Can you work these out from the model? Positions are in its coordinate system, mm. Face numbers are marked on the shaded views. A direction names the side the tool comes from. Round coordinates to 2 decimals unless told otherwise and drop trailing zeros. Loops run counter-clockwise (first coordinate to the right, second up) from the corner with the lowest first, then second, coordinate; pieces in that order, holes last. Notation, with made-up numbers: (50.5, -26) -> (105.5, -26) arc R25 ccw to (105.5, -3) -> close; hole circle Ø6 at (-19, 1). An arc over 180 degrees is marked (long way). Write item = value, one per line.
from build123d import *

# Parameters (mm, degrees)
F1_DEPTH = 5
F2_R     = 1
F3_DEPTH = 25
F4_R     = 1
F5_DEPTH = 25
F6_R     = 4.99999
F7_R     = 5


# Not quite as in the source:
# - a fillet or chamfer is up to 0.001 mm smaller than in the source, because OpenCascade refuses the exact size
# - a feature names something its author has since deleted; it is built from what else it names


with BuildPart() as f1:
    # F0 (on Front) → F1 (new body, symmetric)
    with BuildSketch(Plane.XZ):
        with BuildLine():
            ThreePointArc((3.9053168747, -3.2800152603), (2.1542889978, -4.62266578), (0, -5.1))
            Line((0, -5.1), (0, -8))
            ThreePointArc((0, -8), (3.7724872299, -7.0546679653), (6.6534112025, -4.4420850251))
            Line((6.6534112025, -4.4420850251), (3.9053168747, -3.2800152603))
        make_face()
        with BuildLine():
            ThreePointArc((5.0737374807, -0.5169022898), (4.6972920498, -1.9863150301), (3.9053168747, -3.2800152603))
            Line((3.9053168747, -3.2800152603), (6.6534112025, -4.4420850251))
            ThreePointArc((6.6534112025, -4.4420850251), (7.3683012546, -3.1157882825), (7.8218318085, -1.6789720546))
            Line((7.8218318085, -1.6789720546), (5.0737374807, -0.5169022898))
        make_face()
        with BuildLine():
            ThreePointArc((2, 4.6914816423), (4.392181267, 2.5920539573), (5.0737374807, -0.5169022898))
            Line((5.0737374807, -0.5169022898), (7.8218318085, -1.6789720546))
            ThreePointArc((7.8218318085, -1.6789720546), (7.5363895919, 2.683809218), (5, 6.2449979984))
            ThreePointArc((5, 6.2449979984), (3.5795567819, 7.1544932207), (2, 7.7459666924))
            Line((2, 7.7459666924), (2, 4.6914816423))
        make_face()
        with BuildLine():
            ThreePointArc((7.8218318085, -1.6789720546), (7.3683012546, -3.1157882825), (6.6534112025, -4.4420850251))
            Line((6.6534112025, -4.4420850251), (18.8496842561, -9.5994480802))
            Line((18.8496842561, -9.5994480802), (20.018104862, -6.8363351098))
            Line((20.018104862, -6.8363351098), (7.8218318085, -1.6789720546))
        make_face()
        with BuildLine():
            Line((2, 15), (2, 7.7459666924))
            ThreePointArc((2, 7.7459666924), (3.5795567819, 7.1544932207), (5, 6.2449979984))
            Line((5, 6.2449979984), (5, 15))
            Line((5, 15), (2, 15))
        make_face()
    extrude(amount=F1_DEPTH, both=True)

    # F2 (on face) → F3 (cut)
    with BuildSketch(Plane(origin=(0.584210303, 0, 1.3815564852), x_dir=(0.9210376568, 0, -0.3894735353), z_dir=(0.3894735353, 0, 0.9210376568))):
        with Locations((16.1, 0)):
            Circle(F2_R)
    extrude(amount=-F3_DEPTH, mode=Mode.SUBTRACT)

    # F4 (on face) → F5 (cut)
    with BuildSketch(Plane.YZ.offset(5)):
        with Locations((0, 10.6224989992)):
            Circle(F4_R)
    extrude(amount=-F5_DEPTH, mode=Mode.SUBTRACT)

    # F6 (radius 5 in the source; OpenCascade refuses exactly that, so slightly less here)
    f6_edges = [f1.edges().sort_by_distance(p)[0] for p in [
        (19.433895, 5, -8.217892),
        (19.433895, -5, -8.217892),
        (3.5, -5, 15),
        (3.5, 5, 15),
    ]]
    fillet(f6_edges, radius=F6_R)

    # F7
    f7_edges = [f1.edges().sort_by_distance(p)[0] for p in [
        (5, 0, 6.244998),
        (7.821832, 0, -1.678972),
        (6.653411, 0, -4.442085),
    ]]
    fillet(f7_edges, radius=F7_R)

    # F8: F1 across plane


with BuildPart() as f1_1:
    add(f1.part)
    add(f1.part.mirror(Plane.YZ))


solid = f1_1.part
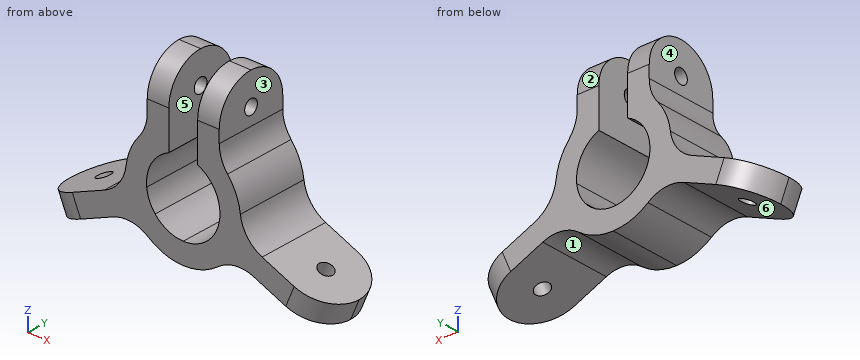
1. Suppose I cut it at B-B, the plane y = 2. List the corners of the cut face in (x, z) for me.
Entries:
outline = (-19.63, -6.67) -> (-18.47, -9.44) -> (-9.79, -5.77) arc R5 cw to (-4.82, -6.38) arc R8 ccw to (4.82, -6.38) arc R5 cw to (9.79, -5.77) -> (18.47, -9.44) -> (19.63, -6.67) -> (10.95, -3) arc R5 cw to (7.94, 0.99) arc R8 ccw to (6.15, 5.11) arc R5 cw to (5, 8.31) -> (5, 14.58) -> (2, 14.58) -> (2, 4.69) arc R5.1 cw (long way) to (-2, 4.69) -> (-2, 14.58) -> (-5, 14.58) -> (-5, 8.31) arc R5 cw to (-6.15, 5.11) arc R8 ccw to (-7.94, 0.99) arc R5 cw to (-10.95, -3) -> close
2. I'm going to push flat-ended pins straight in: pin 1 (6 mm diameter, centred on y = -0.5, z = -1.5, fed in from -X); pin 2 (1.5 mm diameter, centred on y = -3, z = 7, fed in from +X); pin 3 (5 mm diameter, centred on y = 1.5, z = 9, fed in from -X). Where does each tip first touch, or does it pass through?
Entries:
pin_1 = -14.49
pin_2 = 5.44
pin_3 = -5.34
3. For the marked faces 4, 5 and 6, which set-ups out of +Z, -Z, +X, -X, +Y, -Y let a thin tool reach every point of the face, with its end or its side?
Entries:
face_4 = +Z, -X, +Y, -Y
face_5 = +Z, +Y, -Y
face_6 = -Z, +Y, -Y
4. Suppose I cut it at A-A, the plane z = 12.25. List the corners of the cut face in (x, y) for me, and give its area (3 significant figures).
Entries:
outline = (-5, -4.47) -> (-2, -4.47) -> (-2, 4.47) -> (-5, 4.47) -> close; (2, -4.47) -> (5, -4.47) -> (5, 4.47) -> (2, 4.47) -> close
area = 53.6 mm²
5. Suppose I cut it at C-C, the plane z = -2.5. List the corners of the cut face in (x, y) for me, and give its area (3 significant figures).
Entries:
outline = (-10.04, -5) -> (-4.45, -5) -> (-4.45, 5) -> (-10.04, 5) -> close; (4.45, -5) -> (10.04, -5) -> (10.04, 5) -> (4.45, 5) -> close
area = 112 mm²
6. I need wall thicknesses on line 1 (X direction, y = 4, z = -6.75); line 2 (Z direction, x = -2.8, y = 0); line 3 (X direction, y = 3.75, z = 11.5). Which ranges of each line are inside material? Lowest first, please. Write a range as [from, to].
Entries:
line_1 = [-17.88, -12.11], [-4.29, 4.29], [12.11, 17.88]
line_2 = [-7.49, -4.26], [4.26, 9.62], [11.62, 15]
line_3 = [-5, -2], [2, 5]
7. Suppose I cut it at D-D, the plane x = 7. List the corners of the cut face in (y, z) for me, and give its area (3 significant figures).
Entries:
outline = (-5, -5.44) -> (5, -5.44) -> (5, 3.87) -> (-5, 3.87) -> close
area = 93.2 mm²
8. We'd pull the mould along X, two halves only. Please class the marked faces 1, 2 and 3: released by +X, released by -X, zero draft, split by the parting line, or undercut.
Entries:
face_1 = undercut
face_2 = zero draft
face_3 = released by +X
